```python
from build123d import *

# Parameters (mm, degrees)
BOSS_EXTRUDE1_DEPTH = 63.5
SKETCH3_R           = 1.524
BOSS_EXTRUDE2_DEPTH = 7.62
SKETCH4_R           = 2.032
BOSS_EXTRUDE3_DEPTH = 3.81


with BuildPart() as part:
    # Sketch1 → Boss-Extrude1 (new body)
    with BuildSketch(Plane.XY.offset(433.726101294)):
        with BuildLine():
            Line((12.262790096, 63.439286549), (12.817159361, 63.439286549))
            Line((12.817159361, 63.439286549), (13.759849728, 63.439286549))
            ThreePointArc((13.759849728, 63.439286549), (14.295836668, 63.661299609), (14.517849728, 64.197286549))
            Line((14.517849728, 64.197286549), (14.517849728, 67.981786549))
            Line((14.517849728, 67.981786549), (14.517849728, 70.521786549))
            Line((14.517849728, 70.521786549), (-15.788150272, 70.521786549))
            Line((-15.788150272, 70.521786549), (-15.788150272, 72.426786549))
            Line((-15.788150272, 72.426786549), (54.061849728, 72.426786549))
            Line((54.061849728, 72.426786549), (54.061849728, 70.521786549))
            Line((54.061849728, 70.521786549), (23.755849728, 70.521786549))
            Line((23.755849728, 70.521786549), (23.755849728, 67.981786549))
            Line((23.755849728, 67.981786549), (23.755849728, 64.197286549))
            ThreePointArc((23.755849728, 64.197286549), (23.977862788, 63.661299609), (24.513849728, 63.439286549))
            Line((24.513849728, 63.439286549), (28.805849728, 63.439286549))
            Line((28.805849728, 63.439286549), (28.805849728, 59.401079114))
            ThreePointArc((28.805849728, 59.401079114), (28.691364545, 58.825523232), (28.365338327, 58.337590516))
            Line((28.365338327, 58.337590516), (24.822387807, 54.794639996))
            ThreePointArc((24.822387807, 54.794639996), (23.982795062, 54.370887307), (23.055655666, 54.528668358))
            ThreePointArc((23.055655666, 54.528668358), (21.370192512, 55.198240561), (19.580150838, 55.489554446))
            Line((19.580150838, 55.489554446), (19.136849728, 55.179151668))
            Line((19.136849728, 55.179151668), (18.693548619, 55.489554446))
            ThreePointArc((18.693548619, 55.489554446), (16.903506945, 55.198240561), (15.218043791, 54.528668358))
            ThreePointArc((15.218043791, 54.528668358), (14.290904395, 54.370887307), (13.451311649, 54.794639996))
            Line((13.451311649, 54.794639996), (9.908361129, 58.337590516))
            ThreePointArc((9.908361129, 58.337590516), (9.582334911, 58.825523232), (9.467849728, 59.401079114))
            Line((9.467849728, 59.401079114), (9.467849728, 63.439286549))
            Line((9.467849728, 63.439286549), (12.262790096, 63.439286549))
        make_face()
    extrude(amount=-BOSS_EXTRUDE1_DEPTH)

    # Sketch3 → Boss-Extrude2 (add)
    with BuildSketch(Plane(origin=(0, 72.426786549, 0), x_dir=(1, 0, 0), z_dir=(0, 1, 0))):
        with Locations((-0.548150272, -377.554863046)):
            Circle(SKETCH3_R)
        with Locations((50.251849728, -392.794863046)):
            Circle(SKETCH3_R)
        with Locations((50.251849728, -420.734863046)):
            Circle(SKETCH3_R)
        with Locations((-1.818150272, -425.814863046)):
            Circle(SKETCH3_R)
    extrude(amount=BOSS_EXTRUDE2_DEPTH)

    # Sketch4 → Boss-Extrude3 (add)
    with BuildSketch(Plane(origin=(0, 72.426786549, 0), x_dir=(1, 0, 0), z_dir=(0, 1, 0))):
        with Locations((-0.548150272, -377.554863046)):
            Circle(SKETCH4_R)
        with Locations((50.251849728, -392.794863046)):
            Circle(SKETCH4_R)
        with Locations((50.251849728, -420.734863046)):
            Circle(SKETCH4_R)
        with Locations((-1.818150272, -425.814863046)):
            Circle(SKETCH4_R)
    extrude(amount=BOSS_EXTRUDE3_DEPTH)


solid = part.part
```
Can you work these out from the model? Positions are in its coordinate system, mm. A direction names the side the tool comes from. Coordinates: 2 decimals unless noted, no trailing zeros. Loops run counter-clockwise (first coordinate to the right, second up) from the corner with the lowest first, then second, coordinate; pieces in that order, holes last.
Item 1: Suppose I cut it at A-A (z = 412.5). Please give me the cut outline in (x, y).
Answers below:
outline: (-15.79, 70.52) - (14.52, 70.52) - (14.52, 64.2) arc R0.76 cw to (13.76, 63.44) - (9.47, 63.44) - (9.47, 59.4) arc R1.5 ccw to (9.91, 58.34) - (13.45, 54.79) arc R1.5 ccw to (15.22, 54.53) arc R8.38 cw to (18.69, 55.49) - (19.14, 55.18) - (19.58, 55.49) arc R8.38 cw to (23.06, 54.53) arc R1.5 ccw to (24.82, 54.79) - (28.37, 58.34) arc R1.5 ccw to (28.81, 59.4) - (28.81, 63.44) - (24.51, 63.44) arc R0.76 cw to (23.76, 64.2) - (23.76, 70.52) - (54.06, 70.52) - (54.06, 72.43) - (-15.79, 72.43) - close
Item 2: Suppose I cut it at B-B (y = 73.25). Please give me the cut outline in (x, z), then the cut area to 3 significant figures.
Answers below:
outline: circle Ø4.06 at (-1.82, 425.81); circle Ø4.06 at (-0.55, 377.55); circle Ø4.06 at (50.25, 392.79); circle Ø4.06 at (50.25, 420.73)
area: 51.9 mm2
Item 3: Suppose I cut it at C-C (x = 34). Please give me the cut outline in (y, z), then the cut area to 3 significant figures.
Answers below:
outline: (70.52, 370.23) - (72.43, 370.23) - (72.43, 433.73) - (70.52, 433.73) - close
area: 121 mm2
Item 4: I'm going to push flat-ended pins straight in: pin 1 (24 mm diameter, centred on x = -3, z = 407, fed in from -Y); pin 2 (2 mm diameter, centred on x = 20.5, z = 407.5, fed in from -Y); pin 3 (19 mm diameter, centred on x = 34.5, z = 417.5, fed in from +Y). Where does each tip first touch, or does it pass through?
Answers below:
pin 1: stops at y = 70.52
pin 2: stops at y = 55.16
pin 3: stops at y = 72.43
Item 5: Which directions (+Z, -Z, +X, -X, +Y, -Y) give clear straight access to the entire face, cutting with the end or side of a thin tool? Please do faces 4 (the face through (28.806, 61, 402)), 5 (the face through (0.155, 78.115, 378.907)), 6 (the face through (16.928, 55.205, 402.421)), 7 (the face through (23.756, 67, 402)), 8 (the face through (19, 66, 370.226)).
Answers below:
face 4: +Z, -Z, +X, -Y
face 5: +Y
face 6: +Z, -Z, -Y
face 7: +Z, -Z, +X
face 8: -Z, +X, -X, +Y, -Y
Item 6: If we mould it in two halves opening along Y, with no side actions, what happens to faces 1 (the face through (-2.26, 74.31, 427.8)), 2 (the face through (21.395, 55.191, 402.421)), 3 (the face through (12, 63.439, 402))? For each: released by +Y, released by -Y, zero draft, split by the parting line, or undercut.
Answers below:
face 1: zero draft
face 2: released by -Y
face 3: undercut
Item 7: Please list where these lines run through material, in increasing order: L1, parallel to Y at x = 7.5, z = 402; L2, parallel to Y at x = 11.5, z = 420; L3, parallel to X at y = 69.75, z = 413.5.
Answers below:
L1: y = 70.52 to 72.43
L2: y = 56.75 to 63.44, 70.52 to 72.43
L3: x = 14.52 to 23.76
Item 8: Suppose I cut it at D-D (y = 61.25). Please give me the cut outline in (x, z).
Answers below:
outline: (9.47, 370.23) - (28.81, 370.23) - (28.81, 433.73) - (9.47, 433.73) - close
